from build123d import *

# Parameters (mm, degrees)
F2_SIZE  = 0.7
F4_DEPTH = 2
F5_R     = 0.15


with BuildPart() as f1:
    # F0 (on Front) → F1 (revolve)
    with BuildSketch(Plane.XZ):
        Polygon((-2, 10.25), (-2, 0), (0, 0), (0, 12), (-3.75, 12), align=None)
    revolve(axis=Axis((0, 0, 15.756099), (0, 0, 1)))

    # F2
    f2_edges = [f1.edges().sort_by_distance(p)[0] for p in [
        (2, 0, 0),
    ]]
    chamfer(f2_edges, length=F2_SIZE)

    # F3 (on face) → F4 (cut)
    with BuildSketch(Plane.XY.offset(12)):
        Polygon((-1.25, 0.721688), (-1.25, -0.721688), (0, -1.443376), (1.25, -0.721688), (1.25, 0.721688), (0, 1.443376), align=None)
    extrude(amount=-F4_DEPTH, mode=Mode.SUBTRACT)

    # F5
    f5_edges = [f1.edges().sort_by_distance(p)[0] for p in [
        (3.75, 0, 12),
    ]]
    fillet(f5_edges, radius=F5_R)


solid = f1.part
CAD build for the part. Positions are in the model's coordinates, mm. A direction names the side the tool comes from. Round coordinates to 2 decimals unless told otherwise and drop trailing zeros. Write each loop counter-clockwise with the first axis right and the second up, starting at its lowest first coordinate (ties: lowest second). Pieces come first, ordered by that corner, then holes. Notation, with made-up numbers: M 37,66.25 L 69,66.25 A16 ccw 69,70.25 Z; hole C 71,6.25 d7. An arc over 180 degrees is marked long. Use a Markdown table: item, result. Add a question column.
1. 3-axis set-ups, long thin cutter, end or side, ignore diameter. For faces 4 (the face through (0, 0, 0)), 5 (the face through (-1.25, 0, 11)): which of +Z, -Z, +X, -X, +Y, -Y reach the whole face in a straight line?
2. Slice it at B-B on z = 6. Give the cut face in (x, y), then the cut area to 3 significant figures.
3. Slice it at A-A on y = 0. Give the cut face in (x, z), then the cut area to 3 significant figures.
4. Flat gauge pins, fed straight in: P1, Ø0.8, axis at x = 0, y = 0.5, coming from the +Z side; P2, Ø2, axis at y = 1.5, z = 7, coming from the -X side; P3, Ø1.6, axis at y = 0.5, z = 10.5, coming from the +X side. Where does each tip first touch, or does it go through?
5. Pull direction X, two halves, no side cores. Call faces 1 (the face through (0.63, 1.08, 11.01)), 2 (the face through (1.5, 0, 12)), 3 (the face through (0, 2, 5)): released by +X, released by -X, zero draft, split by the parting line, or undercut.
6. Drill centre lines: probe 1 along Z at (x, y) = (-0.5, 0); probe 2 along Y at (x, z) = (-1, 11.75); probe 3 along X at (y, z) = (0, 7.25). Where is each one in solid material? Low to high.
Reply:
| question | item | result |
|---|---|---|
| 1 | face 4 | -Z, +X, -X, +Y, -Y |
| 1 | face 5 | +Z |
| 2 | outline | C 0,0 d4 |
| 2 | area | 12.6 mm^2 |
| 3 | outline | M -3.49,11.74 L -2,10.25 L -2,0.7 L -1.3,0 L 1.3,0 L 2,0.7 L 2,10.25 L 3.49,11.74 A0.15 ccw 3.39,12 L 1.25,12 L 1.25,10 L -1.25,10 L -1.25,12 L -3.39,12 A0.15 ccw Z |
| 3 | area | 45.5 mm^2 |
| 4 | P1 | stops at z = 10 |
| 4 | P2 | stops at x = -1.94 |
| 4 | P3 | stops at x = 3.02 |
| 5 | face 1 | undercut |
| 5 | face 2 | zero draft |
| 5 | face 3 | split by the parting line |
| 6 | probe 1 | z = 0 to 10 |
| 6 | probe 2 | y = -3.35 to -0.87, 0.87 to 3.35 |
| 6 | probe 3 | x = -2 to 2 |
